```python
from build123d import *

# Parameters (mm, degrees)
ESQUISSE1_W             = 100
ESQUISSE1_H             = 100
BOSS_EXTRU_1_DEPTH      = 3
ESQUISSE2_W             = 100
ESQUISSE2_H             = 100
ESQUISSE2_W_2           = 94
ESQUISSE2_H_2           = 94
BOSS_EXTRU_2_DEPTH      = 94
ESQUISSE3_W             = 100
ESQUISSE3_H             = 100
BOSS_EXTRU_3_DEPTH      = 3
ESQUISSE4_W             = 24
ESQUISSE4_H             = 72
ENL_V_MAT_EXTRU_1_DEPTH = 3
CHANFREIN1_SIZE         = 2


with BuildPart() as part:
    # Esquisse1 → Boss.-Extru.1 (new body)
    with BuildSketch(Plane.XY):
        with Locations((50, 50)):
            Rectangle(ESQUISSE1_W, ESQUISSE1_H)
    extrude(amount=BOSS_EXTRU_1_DEPTH)

    # Esquisse2 → Boss.-Extru.2 (add)
    with BuildSketch(Plane.XY.offset(3)):
        with Locations((50, 50)):
            Rectangle(ESQUISSE2_W, ESQUISSE2_H)
        with Locations((50, 50)):
            Rectangle(ESQUISSE2_W_2, ESQUISSE2_H_2, mode=Mode.SUBTRACT)
    extrude(amount=BOSS_EXTRU_2_DEPTH)

    # Esquisse3 → Boss.-Extru.3 (add)
    with BuildSketch(Plane.XY.offset(97)):
        with Locations((50, 50)):
            Rectangle(ESQUISSE3_W, ESQUISSE3_H)
    extrude(amount=BOSS_EXTRU_3_DEPTH)

    # Esquisse4 → Enlèv. mat.-Extru.1 (cut)
    with BuildSketch(Plane(origin=(100, 0, 0), x_dir=(0, 0, -1), z_dir=(1, 0, 0))):
        with Locations((-27, 50)):
            Rectangle(ESQUISSE4_W, ESQUISSE4_H)
    extrude(amount=-ENL_V_MAT_EXTRU_1_DEPTH, mode=Mode.SUBTRACT)

    # Chanfrein1
    chanfrein1_edges = [part.edges().sort_by_distance(p)[0] for p in [
        (50, 100, 0),
        (100, 50, 0),
        (100, 100, 50),
    ]]
    chamfer(chanfrein1_edges, length=CHANFREIN1_SIZE)


solid = part.part
```
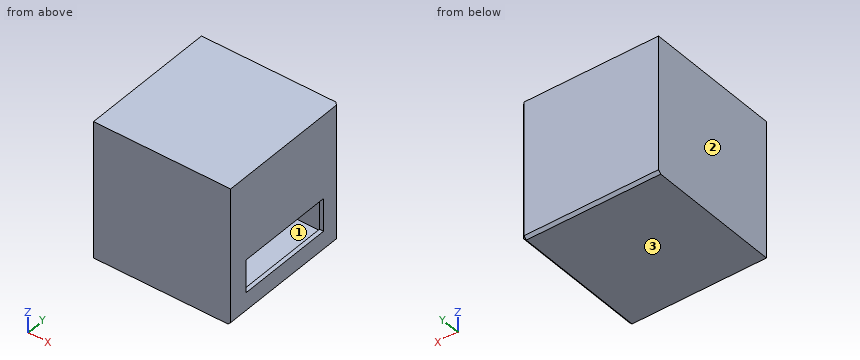
CAD build for the part. Positions are in the model's coordinates, mm. Face numbers are marked on the shaded views. Round coordinates to 2 decimals unless told otherwise and drop trailing zeros. Order: outer loops, then holes, each group sorted by start corner. A loop starts at its lowest first (then second) coordinate and runs counter-clockwise, first axis right, second up.
Item 1: Mould opens along X. For the marked faces 1, 2 and 3 say: pulls with the +X half, pulls with the -X half, needs draft (parallel to the pull), parting line crosses it, or undercut.
Item 2: Saw through at A-A on y = 89.5. Write the cut outline in (x, z), then the cut area to 3 significant figures.
Item 3: Probe line 1 along Z through (x, y) = (44.5, 30). List the from-to ranges inside material, lowest first.
Item 4: Saw through at D-D on y = 22. Write the cut outline in (x, z), then the cut area to 3 significant figures.
Item 5: Saw through at C-C on z = 32. Write the cut outline in (x, y).
Item 6: Pin check, flat tips, straight feed: pin 1 (1.5 mm diameter, centred on x = 98, z = 26, fed in from -Y); pin 2 (1.5 mm diameter, centred on y = 62, z = 36, fed in from +X). Stop position of each tip, or through.
Reported:
1. face 1: undercut
1. face 2: pulls with the -X half
1. face 3: needs draft
2. outline: (0, 0) - (98, 0) - (100, 2) - (100, 100) - (0, 100) - close; hole (3, 3) - (97, 3) - (97, 97) - (3, 97) - close
2. area: 1,160 mm2
3. line 1: z = 0 to 3, 97 to 100
4. outline: (0, 0) - (98, 0) - (100, 2) - (100, 15) - (97, 15) - (97, 3) - (3, 3) - (3, 97) - (97, 97) - (97, 39) - (100, 39) - (100, 100) - (0, 100) - close
4. area: 1,090 mm2
5. outline: (0, 0) - (100, 0) - (100, 14) - (97, 14) - (97, 3) - (3, 3) - (3, 97) - (97, 97) - (97, 86) - (100, 86) - (100, 98) - (98, 100) - (0, 100) - close
6. pin 1: stops at y = 0
6. pin 2: stops at x = 3
